```python
from build123d import *

# Parameters (mm, degrees)
SKETCH2_R           = 15
BOSS_EXTRUDE1_DEPTH = 230
CUT_EXTRUDE1_START  = -160
SKETCH3_R           = 15
SKETCH3_R_2         = 13
CUT_EXTRUDE1_DEPTH  = 160
CUT_EXTRUDE3_START  = -75
SKETCH4_R           = 13
SKETCH4_R_2         = 11.5
CUT_EXTRUDE3_DEPTH  = 75
CUT_EXTRUDE4_START  = -40
SKETCH5_R           = 11.5
SKETCH5_R_2         = 10.5
CUT_EXTRUDE4_DEPTH  = 40
SKETCH6_R           = 15
SKETCH6_R_2         = 11.5
CUT_EXTRUDE5_DEPTH  = 30
BOSS_EXTRUDE2_DEPTH = 40


with BuildPart() as part:
    # Sketch2 → Boss-Extrude1 (new body)
    with BuildSketch(Plane.XY):
        Circle(SKETCH2_R)
    extrude(amount=BOSS_EXTRUDE1_DEPTH)

    # Sketch3 → Cut-Extrude1 (cut)
    with BuildSketch(Plane.XY.offset(230).offset(CUT_EXTRUDE1_START)):
        Circle(SKETCH3_R)
        Circle(SKETCH3_R_2, mode=Mode.SUBTRACT)
    extrude(amount=CUT_EXTRUDE1_DEPTH, mode=Mode.SUBTRACT)

    # Sketch4 → Cut-Extrude3 (cut)
    with BuildSketch(Plane.XY.offset(230).offset(CUT_EXTRUDE3_START)):
        Circle(SKETCH4_R)
        Circle(SKETCH4_R_2, mode=Mode.SUBTRACT)
    extrude(amount=CUT_EXTRUDE3_DEPTH, mode=Mode.SUBTRACT)

    # Sketch5 → Cut-Extrude4 (cut)
    with BuildSketch(Plane.XY.offset(230).offset(CUT_EXTRUDE4_START)):
        Circle(SKETCH5_R)
        Circle(SKETCH5_R_2, mode=Mode.SUBTRACT)
    extrude(amount=CUT_EXTRUDE4_DEPTH, mode=Mode.SUBTRACT)

    # Sketch6 → Cut-Extrude5 (cut)
    with BuildSketch(Plane(origin=(0, 0, 0), x_dir=(-1, 0, 0), z_dir=(0, 0, -1))):
        Circle(SKETCH6_R)
        with Locations(Location((0, 0, 0), (0, 0, 180))):
            Circle(SKETCH6_R_2, mode=Mode.SUBTRACT)
    extrude(amount=-CUT_EXTRUDE5_DEPTH, mode=Mode.SUBTRACT)

    # Sketch8 → Boss-Extrude2 (add)
    with BuildSketch(Plane.XY.offset(70)):
        with BuildLine():
            Line((-6, 16), (6, 16))
            Line((6, 16), (6, 11.532562595))
            ThreePointArc((6, 11.532562595), (0, 13), (-6, 11.532562595))
            Line((-6, 11.532562595), (-6, 16))
        make_face()
    extrude(amount=BOSS_EXTRUDE2_DEPTH)


solid = part.part
```
Check sheet for the modelled part. Datum: model origin and axes. Units: mm. A direction names the side the tool comes from. Give positions to 0.01 mm unless a question says otherwise; leave off trailing zeros. Order: outer loops, then holes, each group sorted by start corner. A loop starts at its lowest first (then second) coordinate and runs counter-clockwise, first axis right, second up. Notation, with made-up numbers: (6, 21) -> (49, 21) arc R5 ccw to (49, 27) -> close; hole circle Ø11 at (-20, 58). An arc over 180 degrees is marked (long way). Return JSON: item names as keys, results as strings.
1. Set-up check for faces 1 (the flat face through (0, 0, 0)), 2 (the cylindrical face through (10, 3.2, 209.7)), 3 (the cylindrical face through (-1.5, -11.4, 14.8)), 4 (the flat face through (-6, 14, 90)), 5 (the flat face through (6, 14, 90)): record each of +Z, -Z, +X, -X, +Y, -Y from which the full face is reachable in a straight line by a thin tool's end or side.
From the geometry:
{"face 1": "-Z, +X, -X, +Y, -Y", "face 2": "+Z", "face 3": "-Z", "face 4": "+Z, -X, +Y", "face 5": "+Z, +X, +Y"}
2. Cross-section at C-C, the plane z = 193.5. Record the cut outline in (x, y), plus the area to 3 significant figures.
From the geometry:
{"outline": "circle Ø21 at (0, 0)", "area": "346 mm^2"}
3. Cross-section at B-B, the plane y = 0. Record the cut outline in (x, z).
From the geometry:
{"outline": "(-15, 30) -> (-11.5, 30) -> (-11.5, 0) -> (11.5, 0) -> (11.5, 30) -> (15, 30) -> (15, 70) -> (13, 70) -> (13, 155) -> (11.5, 155) -> (11.5, 190) -> (10.5, 190) -> (10.5, 230) -> (-10.5, 230) -> (-10.5, 190) -> (-11.5, 190) -> (-11.5, 155) -> (-13, 155) -> (-13, 70) -> (-15, 70) -> close"}
4. Material ranges on probe 1 along Z at (x, y) = (-13, -2); probe 2 along Z at (x, y) = (-11, -5); probe 3 along X at (y, z) = (1, 83.5), recorded low to high. Write a range as [from, to].
From the geometry:
{"probe 1": "[30, 70]", "probe 2": "[30, 155]", "probe 3": "[-12.96, 12.96]"}
5. Go/stop test with flat-tipped pins: P1, Ø1.8, axis at x = -0.5, y = 15, coming from the -Z side; P2, Ø1.5, axis at x = -6, y = -4.5, coming from the -Z side; P3, Ø2, axis at x = -2, y = 14, coming from the +Z side; P4, Ø10, axis at y = -8, z = 202, coming from the -X side. Record where each tip stops, or that it passes through.
From the geometry:
{"P1": "z = 30", "P2": "z = 0", "P3": "z = 110", "P4": "x = -10.06"}
6. Cross-section at D-D, the plane y = 8.5. Record the cut outline in (x, z).
From the geometry:
{"outline": "(-12.36, 30) -> (-7.75, 30) -> (-7.75, 0) -> (7.75, 0) -> (7.75, 30) -> (12.36, 30) -> (12.36, 70) -> (9.84, 70) -> (9.84, 155) -> (7.75, 155) -> (7.75, 190) -> (6.16, 190) -> (6.16, 230) -> (-6.16, 230) -> (-6.16, 190) -> (-7.75, 190) -> (-7.75, 155) -> (-9.84, 155) -> (-9.84, 70) -> (-12.36, 70) -> close"}
7. Cross-section at A-A, the plane x = 0. Record the cut outline in (y, z), plus the area to 4 significant figures.
From the geometry:
{"outline": "(-15, 30) -> (-11.5, 30) -> (-11.5, 0) -> (11.5, 0) -> (11.5, 30) -> (15, 30) -> (15, 70) -> (16, 70) -> (16, 110) -> (13, 110) -> (13, 155) -> (11.5, 155) -> (11.5, 190) -> (10.5, 190) -> (10.5, 230) -> (-10.5, 230) -> (-10.5, 190) -> (-11.5, 190) -> (-11.5, 155) -> (-13, 155) -> (-13, 70) -> (-15, 70) -> close", "area": "5,865 mm^2"}
